The listing builds one solid part. Answer for the finished solid, in the listing's coordinates (mm). Face numbers are marked on the shaded views. A direction names the side the tool comes from. Coordinates: 2 decimals unless noted, no trailing zeros. Loops run counter-clockwise (first coordinate to the right, second up) from the corner with the lowest first, then second, coordinate; pieces in that order, holes last. Notation, with made-up numbers: (24.5, 61) - (37.5, 61) arc R33 cw to (37.5, 97) - close; hole circle Ø11 at (6.5, 47.5). An arc over 180 degrees is marked (long way). Put each result on its own line as item: value.
```python
from build123d import *

# Parameters (mm, degrees)
SKETCH1_W           = 5
SKETCH1_H           = 5
BOSS_EXTRUDE1_DEPTH = 5
CUT_EXTRUDE2_DEPTH  = 2
CUT_EXTRUDE3_DEPTH  = 2
CUT_EXTRUDE4_DEPTH  = 2
SKETCH6_W           = 3
SKETCH6_H           = 2
CUT_EXTRUDE5_DEPTH  = 1
CUT_EXTRUDE6_DEPTH  = 1
CUT_EXTRUDE7_DEPTH  = 1
CUT_EXTRUDE8_DEPTH  = 3


with BuildPart() as part:
    # Sketch1 → Boss-Extrude1 (new body)
    with BuildSketch(Plane.XY):
        Rectangle(SKETCH1_W, SKETCH1_H)
    extrude(amount=BOSS_EXTRUDE1_DEPTH)

    # Sketch3 → Cut-Extrude2 (cut)
    with BuildSketch(Plane(origin=(0, 2.5, 0), x_dir=(1, 0, 0), z_dir=(0, 1, 0))):
        Polygon((-2.5, -5), (-2.5, -3.999504656), (-0.5, -3.999504656), (-0.5, -3), (0.5, -3), (0.5, -1), (2.5, -1), (2.5, -5), align=None)
    extrude(amount=-CUT_EXTRUDE2_DEPTH, mode=Mode.SUBTRACT)

    # Sketch4 → Cut-Extrude3 (cut)
    with BuildSketch(Plane(origin=(-0.5, 0, 0), x_dir=(0, 0, -1), z_dir=(1, 0, 0))):
        Polygon((-3, 2.5), (-3.999504656, 0.5), (-3.999504656, 2.5), align=None)
    extrude(amount=-CUT_EXTRUDE3_DEPTH, mode=Mode.SUBTRACT)

    # Sketch5 → Cut-Extrude4 (cut)
    with BuildSketch(Plane.XY.offset(1)):
        Polygon((0.5, 2.5), (2.5, 0.5), (2.5, 2.5), align=None)
    extrude(amount=-CUT_EXTRUDE4_DEPTH, mode=Mode.SUBTRACT)

    # Sketch6 → Cut-Extrude5 (cut)
    with BuildSketch(Plane.XY.offset(5)):
        with Locations((1, -0.5)):
            Rectangle(SKETCH6_W, SKETCH6_H)
    extrude(amount=-CUT_EXTRUDE5_DEPTH, mode=Mode.SUBTRACT)

    # Sketch7 → Cut-Extrude6 (cut)
    with BuildSketch(Plane.XY.offset(4)):
        Polygon((2.5, 0.5), (0.5, 0.5), (2.5, -1.5), align=None)
    extrude(amount=-CUT_EXTRUDE6_DEPTH, mode=Mode.SUBTRACT)

    # Sketch11 → Cut-Extrude7 (cut)
    with BuildSketch(Plane(origin=(1.222222222, 0.611111111, 1.222222222), x_dir=(0.745355992, -0.298142397, -0.596284794), z_dir=(0.666666667, 0.333333333, 0.666666667))):
        Polygon((-0.96896279, 1.788854382), (-3.652244363, 0.894427191), (-3.652244363, -1.341419262), (-0.96896279, -0.447213595), align=None)
    extrude(amount=CUT_EXTRUDE7_DEPTH, mode=Mode.SUBTRACT)

    # Sketch12 → Cut-Extrude8 (cut, through all)
    with BuildSketch(Plane(origin=(0, 0.5, 0), x_dir=(1, 0, 0), z_dir=(0, 1, 0))):
        Polygon((0.5, -2), (-1.5, -3.999504656), (0.5, -4), align=None)
    extrude(amount=CUT_EXTRUDE8_DEPTH, mode=Mode.SUBTRACT)


solid = part.part
```
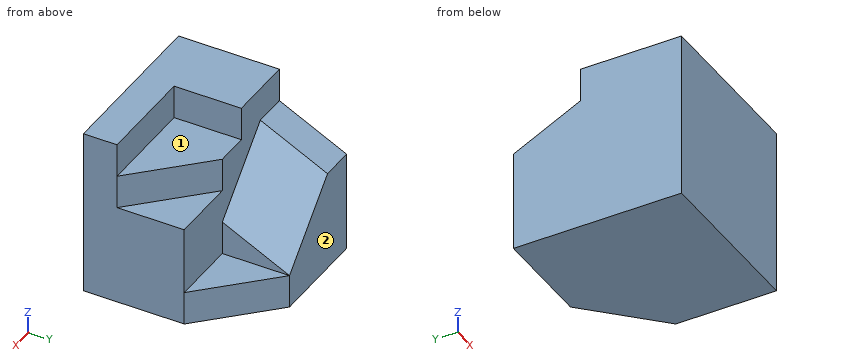
1) Each of these flat-tipped pins is pushed along its axis until it touches: pin 1 (1.6 mm diameter, centred on x = 1.5, y = -0.5, fed in from +Z); pin 2 (0.8 mm diameter, centred on y = 1.5, z = 1.5, fed in from +X); pin 3 (0.5 mm diameter, centred on x = 1.5, z = 4.5, fed in from +Y). Where does it stop, or does it pass through?
Found:
pin 1: stops at z = 4
pin 2: stops at x = 0.5
pin 3: stops at y = -1.5
2) The part is cut by section B-B (z = 1.8). Give the vertices of the cut face in (x, y), and give its area (3 significant figures).
Found:
outline: (-2.5, -2.5) - (2.5, -2.5) - (2.5, 0.5) - (0.5, 0.5) - (0.5, 0.9) - (-0.3, 2.5) - (-2.5, 2.5) - close
area: 20.4 mm^2
3) The part is cut by section C-C (y = -0.6). Give the vertices of the cut face in (x, z), and give its area (3 significant figures).
Found:
outline: (-2.5, 0) - (2.5, 0) - (2.5, 3) - (1.6, 3) - (1.6, 4) - (-0.5, 4) - (-0.5, 5) - (-2.5, 5) - close
area: 21.1 mm^2
4) The part is cut by section D-D (y = 0.25). Give the vertices of the cut face in (x, z).
Found:
outline: (-2.5, 0) - (2.5, 0) - (2.5, 3) - (0.75, 3) - (0.75, 4) - (-0.5, 4) - (-0.5, 5) - (-2.5, 5) - close
5) Straight lines are drawn through the part: L1, parallel to Z at x = 0.75, y = 0.3; L2, parallel to Z at x = -0.4, y = -0.4; L3, parallel to Y at x = 2.1, z = 2.35. For each, find the intervals that lie inside material, in ascending order. Write a range as [from, to].
Found:
L1: z = [0, 3]
L2: z = [0, 4]
L3: y = [-2.5, 0.5]
6) For the marked faces 1 and 2, determine the directions among +Z, -Z, +X, -X, +Y, -Y from which every point of the face is accessible in a straight line to the end or side of a thin tool.
Found:
face 1: +Z, +X, +Y
face 2: +Z, -Z, +X, -X, +Y
7) The part is cut by section A-A (x = 2.2). Give the vertices of the cut face in (y, z), and give its area (3 significant figures).
Found:
outline: (-2.5, 0) - (0.8, 0) - (0.8, 1) - (0.5, 1) - (0.5, 3) - (-1.2, 3) - (-1.2, 4) - (-1.5, 4) - (-1.5, 5) - (-2.5, 5) - close
area: 11.6 mm^2
